Read the model definition and answer for the solid it produces. Units are mm, in the model's axes. Face numbers are marked on the shaded views. A direction names the side the tool comes from. Coordinates: 2 decimals unless noted, no trailing zeros. Write each loop counter-clockwise with the first axis right and the second up, starting at its lowest first coordinate (ties: lowest second). Pieces come first, ordered by that corner, then holes. Notation, with made-up numbers: (9, 57.25) -> (21, 57.25) arc R24 ccw to (21, 69.25) -> close; hole circle Ø3 at (48.5, 71.5). An arc over 180 degrees is marked (long way). One line per item, written item: value. Start each with the question number.
1. Given P1, Ø12, axis at x = -21.5, y = 17, coming from the +Z side; P2, Ø1, axis at x = 13.5, y = 7.5, coming from the +Z side; P3, Ø8, axis at x = -12, y = 4, coming from the -Z side, each flat-ended and moving along its own axis, determine where each tip first touches the part or whether it passes through.
2. For the marked faces 1 and 2, determine the directions among +Z, -Z, +X, -X, +Y, -Y from which every point of the face is accessible in a straight line to the end or side of a thin tool.
3. Find section C-C, the plane y = 16. Write down the section's boundary in (x, z).
4. Find section A-A, the plane x = 20. State how many separate pieces and enclosed holes the cut face has, and give its area (3 significant figures).
5. Consider line 1 along Y through (x, z) = (23, 13.5); line 2 along Y through (x, z) = (20, -10); line 3 along Z through (x, y) = (19, 22.25). Determine where each line is inside the solid, lowest interval first.
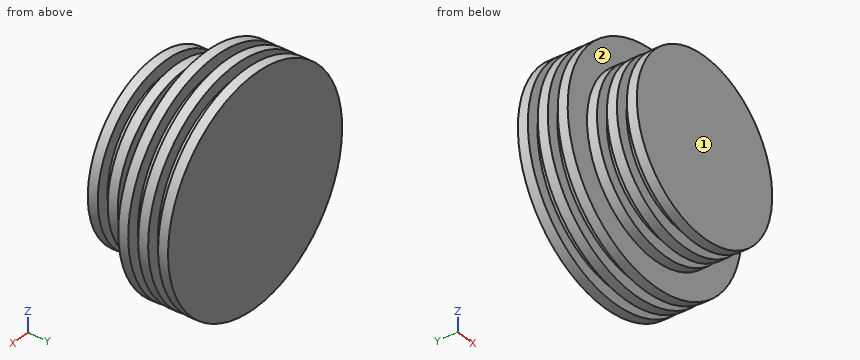
```python
from build123d import *

# Parameters (mm, degrees)
SKETCH1_R           = 22.225
SKETCH1_R_2         = 19.05
BOSS_EXTRUDE1_DEPTH = 2.54
SKETCH3_R           = 19.05
BOSS_EXTRUDE2_DEPTH = 12.7
LPATTERN1_COUNT     = 3
LPATTERN1_PITCH     = 5.08
SKETCH5_R           = 25.4
SKETCH5_R_2         = 22.225
BOSS_EXTRUDE3_DEPTH = 12.7
SKETCH7_R           = 28.575
BOSS_EXTRUDE4_DEPTH = 2.54
LPATTERN2_COUNT     = 3
LPATTERN2_PITCH     = 5.08


with BuildPart() as part:
    # Sketch1 → Boss-Extrude1 (new body)
    with BuildSketch(Plane(origin=(0, 0, 0), x_dir=(1, 0, 0), z_dir=(0, 1, 0))):
        with Locations(Location((0, 0, 0), (0, 0, 270))):
            Circle(SKETCH1_R)
        with Locations(Location((0, 0, 0), (0, 0, 270))):
            Circle(SKETCH1_R_2, mode=Mode.SUBTRACT)
    boss_extrude1 = extrude(amount=BOSS_EXTRUDE1_DEPTH)

    # Sketch3 → Boss-Extrude2 (add)
    with BuildSketch(Plane.XZ):
        with Locations(Location((0, 0, 0), (0, 0, 270))):
            Circle(SKETCH3_R)
    extrude(amount=-BOSS_EXTRUDE2_DEPTH)

    # LPattern1: Boss-Extrude1 ×3
    with Locations(*[(0, i * LPATTERN1_PITCH, 0) for i in range(1, LPATTERN1_COUNT)]):
        add(boss_extrude1)

    # Sketch5 → Boss-Extrude3 (add)
    # profile 1 of 2: a face of its own
    with BuildSketch(Plane(origin=(0, 12.7, 0), x_dir=(1, 0, 0), z_dir=(0, 1, 0))):
        with Locations(Location((0, 0, 0), (0, 0, 270))):
            Circle(SKETCH5_R)
        with Locations(Location((0, 0, 0), (0, 0, 270))):
            Circle(SKETCH5_R_2, mode=Mode.SUBTRACT)
    # profile 2 of 2: a face of its own
    with BuildSketch(Plane(origin=(0, 12.7, 0), x_dir=(1, 0, 0), z_dir=(0, 1, 0))):
        with Locations(Location((0, 0, 0), (0, 0, 270))):
            Circle(SKETCH5_R_2)
    extrude(amount=BOSS_EXTRUDE3_DEPTH)

    # Sketch7 → Boss-Extrude4 (add)
    with BuildSketch(Plane.XZ.offset(-12.7)):
        with Locations(Location((0, 0, 0), (0, 0, 270))):
            Circle(SKETCH7_R)
    boss_extrude4 = extrude(amount=-BOSS_EXTRUDE4_DEPTH)

    # LPattern2: Boss-Extrude4 ×3
    with Locations(*[(0, i * LPATTERN2_PITCH, 0) for i in range(1, LPATTERN2_COUNT)]):
        add(boss_extrude4)


solid = part.part
```
Answer block:
1. P1: stops at z = 23.97
1. P2: stops at z = 18.03
1. P3: stops at z = -20.68
2. face 1: +Z, -Z, +X, -X, -Y
2. face 2: -Y
3. outline: circle Ø50.8 at (0, 0)
4. separate pieces: 3
4. enclosed holes: 0
4. area: 618 mm2
5. line 1: y = 12.7 to 15.24, 17.78 to 20.32, 22.86 to 25.4
5. line 2: y = 12.7 to 25.4
5. line 3: z = -16.86 to 16.86
